```python
from build123d import *

# Parameters (mm, degrees)
F2_R     = 1.25
F3_DEPTH = 5.1


# Not quite as in the source:
# - a feature names something its author has since deleted; it is built from what else it names


with BuildPart() as f1:
    # F0 (on Front) → F1 (revolve)
    with BuildSketch(Plane.XZ):
        with BuildLine():
            Line((0, 1.2750519672), (0, 0))
            Line((0, 0), (13, 0))
            ThreePointArc((13, 0), (14.4142135624, 0.5857864376), (15, 2))
            Line((15, 2), (15, 2.8974551242))
            ThreePointArc((15, 2.8974551242), (14.6395651733, 3.6234077181), (13.8866530545, 3.9234806662))
            Line((13.8866530545, 3.9234806662), (12.773306109, 3.9234806662))
            ThreePointArc((12.773306109, 3.9234806662), (11.3706801368, 3.5459784592), (10.2690433302, 2.5992663167))
            Line((10.2690433302, 2.5992663167), (10.1940094677, 2.4367391619))
            ThreePointArc((10.1940094677, 2.4367391619), (9.4559973183, 1.5903226699), (8.378181381, 1.2750519672))
            Line((8.378181381, 1.2750519672), (0, 1.2750519672))
        make_face()
    revolve(axis=Axis((0, 0, 0.6375259836), (0, 0, -1)))

    # F2 (on face) → F3 (cut)
    with BuildSketch(Plane.XY.offset(1.2750519672)):
        with Locations((3.0000000261, -2.9038460925)):
            Circle(F2_R)
        with Locations((2.9038460925, 3.0000000261)):
            Circle(F2_R)
        with Locations((-3.0000000261, 2.9038460925)):
            Circle(F2_R)
        with Locations((-2.9038460925, -3.0000000261)):
            Circle(F2_R)
    extrude(amount=-F3_DEPTH, mode=Mode.SUBTRACT)


solid = f1.part
```
Check sheet for the modelled part. Datum: model origin and axes. Units: mm. Give positions to 0.01 mm unless a question says otherwise; leave off trailing zeros. Loops run counter-clockwise (first coordinate to the right, second up) from the corner with the lowest first, then second, coordinate; pieces in that order, holes last. Notation, with made-up numbers: (-15.5, 57) - (19.5, 57) arc R31 ccw to (19.5, 81) - close; hole circle Ø7 at (40, 68.25). An arc over 180 degrees is marked (long way). One line per question, with ' | ' between items. Start each with the question number.
1. Cross-section at C-C, the plane z = 0.5. Enter the section's corners in (x, y).
2. Cross-section at A-A, the plane y = 0. Enter the section's corners in (x, z), plus the area to 3 significant figures.
3. Gauge pin test, flat ends, axial feed: pin 1 Ø3 at (x, y) = (-3, 2.9) entering from -Z; pin 2 Ø4 at (x, y) = (2.9, 3) entering from +Z; pin 3 Ø1 at (y, z) = (10.5, 3) entering from +X; pin 4 Ø1.5 at (x, z) = (6.5, 3.5) entering from -Y. Record the tip position at first contact, or that the pin passes through.
4. Draft check along X on faces 1 (the cylindrical face through (-1.81, 3.28, 0.65)), 2 (the flat face through (0, 0, 0)), 3 (the cylindrical face through (-14.985, -0.66, 2.455)), 4 (the flat face through (0, 0, 1.275)). Enter one of: released by +X, released by -X, zero draft, split by the parting line, or undercut.
5. Material ranges on line 1 along X through (y, z) = (-3, 1.05); line 2 along Y through (x, z) = (3, 0.45); line 3 along Y through (x, z) = (-3, 0.3), recorded low to high. Write a range as [from, to].
Check result:
1) outline: circle Ø28.65 at (0, 0); hole circle Ø2.5 at (-3, 2.9); hole circle Ø2.5 at (-2.9, -3); hole circle Ø2.5 at (2.9, 3); hole circle Ø2.5 at (3, -2.9)
2) outline: (-15, 2) arc R2 ccw to (-13, 0) - (13, 0) arc R2 ccw to (15, 2) - (15, 2.9) arc R1.13 ccw to (13.89, 3.92) - (12.77, 3.92) arc R3.28 ccw to (10.27, 2.6) - (10.19, 2.44) arc R2 cw to (8.38, 1.28) - (-8.38, 1.28) arc R2 cw to (-10.19, 2.44) - (-10.27, 2.6) arc R3.28 ccw to (-12.77, 3.92) - (-13.89, 3.92) arc R1.13 ccw to (-15, 2.9) - close | area: 60.3 mm2
3) pin 1: stops at z = 0 | pin 2: stops at z = 1.28 | pin 3: stops at x = 11.17 | pin 4: stops at y = -13.76
4) face 1: undercut | face 2: zero draft | face 3: split by the parting line | face 4: undercut
5) line 1: x = [-14.45, -4.15], [-1.65, 1.75], [4.25, 14.45] | line 2: y = [-13.94, -4.15], [-1.65, 1.75], [4.25, 13.94] | line 3: y = [-13.73, -4.25], [-1.75, 1.65], [4.15, 13.73]
